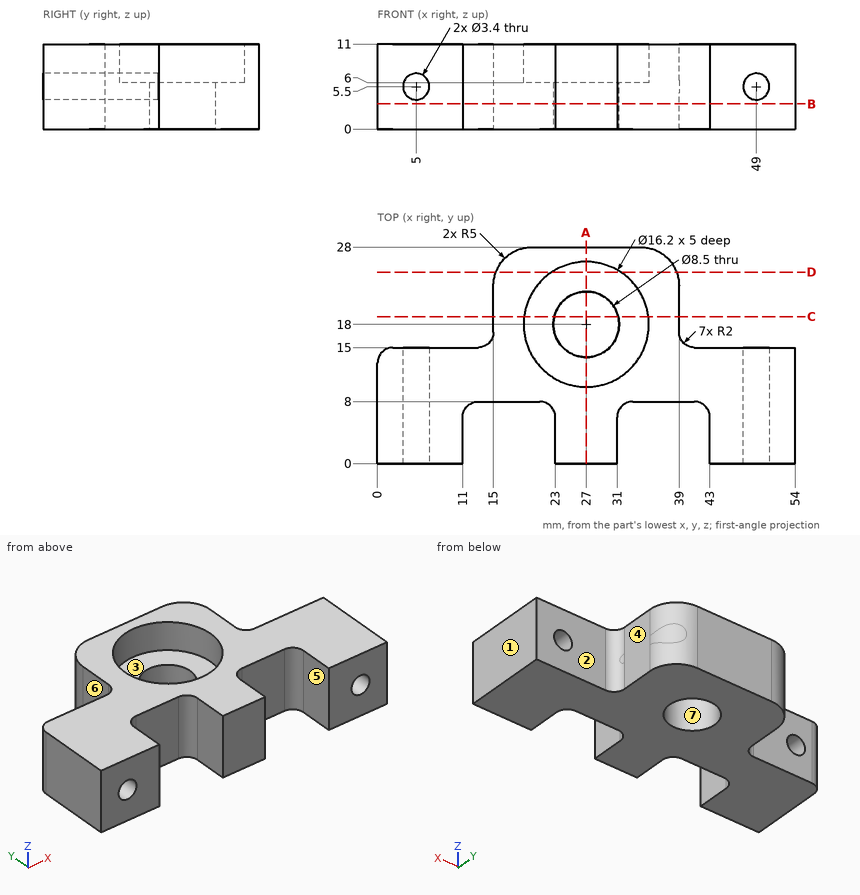
Geometry: see drawing. Coordinates: mm, zero at the bounding-box minimum. A direction names the side the tool comes from. Give positions to 0.01 mm unless a question says otherwise; leave off trailing zeros. Write each loop counter-clockwise with the first axis right and the second up, starting at its lowest first coordinate (ties: lowest second). Pieces come first, ordered by that corner, then holes. Notation, with made-up numbers: (32.25, 63) -> (65.25, 63) arc R26 ccw to (65.25, 79) -> close; hole circle Ø1 at (32.25, 79.25). An arc over 180 degrees is marked (long way). Use one line per item in the form item = value. Start each with the question number.
1) Section query A-A on x = 27. Return the cut outline in (y, z), then the cut area to 3 significant figures.
2) Draft query along X for the marked faces 1, 2 and 3. Return one class per face: pulls with the +X half, pulls with the -X half, needs draft (parallel to the pull), parting line crosses it, or undercut.
3) Section query B-B on z = 3.25. Return the cut outline in (x, y), then the cut area to 3 significant figures.
4) Section query D-D on y = 24.75. Return the cut outline in (x, z).
5) Ray query, probe 1 along X at (y, z) = (6, 2.5); probe 2 along Y at (x, z) = (27, 4.55); probe 3 along Z at (x, y) = (5, 11). Return the intervals inside material, ascending. Write a range as from..to.
6) Pin query (flat end, axial travel): pin 1 (2.5 mm diameter, centred on x = 36, z = 3.5, fed in from -Y); pin 2 (5 mm diameter, centred on y = 19.5, z = 3, fed in from -X); pin 3 (8 mm diameter, centred on x = 26.5, y = 21.5, fed in from +Z). Return the tip coordinate at first contact, or that it passes through.
7) Section query C-C on y = 19. Return the cut outline in (x, z).
8) Set-up query: the marked faces 4, 5, 6 and 7. Return all of +Z, -Z, +X, -X, +Y, -Y with unobstructed straight access to the full face (end or side cutting, diameter ignored); none if empty.
Outcome:
q1.outline = (0, 0) -> (13.75, 0) -> (13.75, 6) -> (9.9, 6) -> (9.9, 11) -> (0, 11) -> close; (22.25, 0) -> (28, 0) -> (28, 11) -> (26.1, 11) -> (26.1, 6) -> (22.25, 6) -> close
q1.area = 176 mm^2
q2.face_1 = pulls with the +X half
q2.face_2 = needs draft
q2.face_3 = undercut
q3.outline = (0, 0) -> (11, 0) -> (11, 6) arc R2 cw to (13, 8) -> (21, 8) arc R2 cw to (23, 6) -> (23, 0) -> (31, 0) -> (31, 6) arc R2 cw to (33, 8) -> (41, 8) arc R2 cw to (43, 6) -> (43, 0) -> (54, 0) -> (54, 15) -> (41, 15) arc R2 cw to (39, 17) -> (39, 23) arc R5 ccw to (34, 28) -> (20, 28) arc R5 ccw to (15, 23) -> (15, 17) arc R2 cw to (13, 15) -> (2, 15) arc R2 ccw to (0, 13) -> close; hole circle Ø8.5 at (27, 18)
q3.area = 867 mm^2
q4.outline = (15.32, 0) -> (38.68, 0) -> (38.68, 11) -> (31.48, 11) -> (31.48, 6) -> (22.52, 6) -> (22.52, 11) -> (15.32, 11) -> close
q5.probe_1 = 0..11, 23..31, 43..54
q5.probe_2 = 0..13.75, 22.25..28
q5.probe_3 = 0..3.8, 7.2..11
q6.pin_1 = 8
q6.pin_2 = 15
q6.pin_3 = 6
q7.outline = (15, 0) -> (22.87, 0) -> (22.87, 6) -> (18.96, 6) -> (18.96, 11) -> (15, 11) -> close; (31.13, 0) -> (39, 0) -> (39, 11) -> (35.04, 11) -> (35.04, 6) -> (31.13, 6) -> close
q8.face_4 = +Z, -Z, +X, +Y
q8.face_5 = +Z, -Z, -Y
q8.face_6 = +Z, -Z, -X, +Y
q8.face_7 = +Z, -Z
